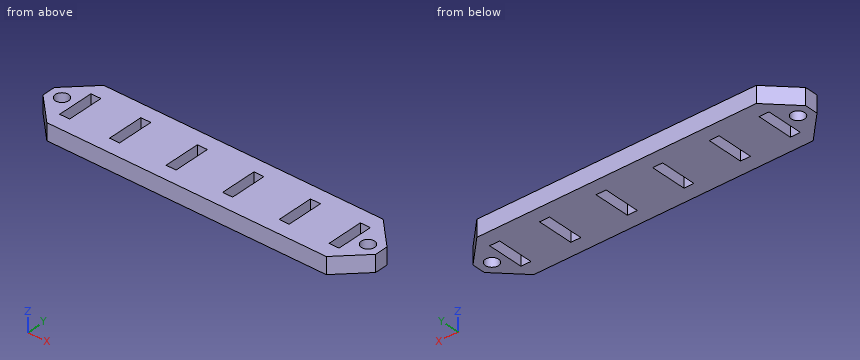
```python
from build123d import *

# Parameters (mm, degrees)
SKETCH1_W           = 100
SKETCH1_H           = 20
BOSS_EXTRUDE1_DEPTH = 5
SKETCH2_R           = 2
SKETCH2_W           = 3
SKETCH2_H           = 11
CUT_EXTRUDE1_DEPTH  = 5
CUT_EXTRUDE2_DEPTH  = 5


with BuildPart() as part:
    # Sketch1 → Boss-Extrude1 (new body)
    with BuildSketch(Plane.XY):
        with Locations((50, 10)):
            Rectangle(SKETCH1_W, SKETCH1_H)
    extrude(amount=BOSS_EXTRUDE1_DEPTH)

    # Sketch2 → Cut-Extrude1 (cut)
    with BuildSketch(Plane(origin=(0, 0, 0), x_dir=(-1, 0, 0), z_dir=(0, 0, -1))):
        with Locations((-96, 10)):
            Circle(SKETCH2_R)
        with Locations((-4, 10)):
            Circle(SKETCH2_R)
        with Locations((-90.5, 10)):
            Rectangle(SKETCH2_W, SKETCH2_H)
        with Locations((-75.5, 10)):
            Rectangle(SKETCH2_W, SKETCH2_H)
        with Locations((-58.5, 10)):
            Rectangle(SKETCH2_W, SKETCH2_H)
        with Locations((-41.5, 10)):
            Rectangle(SKETCH2_W, SKETCH2_H)
        with Locations((-24.5, 10)):
            Rectangle(SKETCH2_W, SKETCH2_H)
        with Locations((-9.5, 10)):
            Rectangle(SKETCH2_W, SKETCH2_H)
    extrude(amount=-CUT_EXTRUDE1_DEPTH, mode=Mode.SUBTRACT)

    # Sketch3 → Cut-Extrude2 (cut)
    with BuildSketch(Plane(origin=(0, 0, 0), x_dir=(-1, 0, 0), z_dir=(0, 0, -1))):
        Polygon((-92, 20), (-100, 12), (-100, 20), align=None)
        Polygon((-100, 8), (-100, 0), (-92, 0), align=None)
        Polygon((-8, 20), (0, 20), (0, 12), align=None)
        Polygon((0, 8), (-8, 0), (0, 0), align=None)
    extrude(amount=-CUT_EXTRUDE2_DEPTH, mode=Mode.SUBTRACT)


solid = part.part
```
For this review, take the finished solid that the model builds, in its own axes (mm). Round coordinates to 2 decimals unless told otherwise and drop trailing zeros. Order: outer loops, then holes, each group sorted by start corner. A loop starts at its lowest first (then second) coordinate and runs counter-clockwise, first axis right, second up.
Q1. We need section A-A, the plane y = 7. Give the boundary of the cut face in (x, z), plus the area to 3 significant figures.
Findings below:
outline: (1, 0) - (8, 0) - (8, 5) - (1, 5) - close; (11, 0) - (23, 0) - (23, 5) - (11, 5) - close; (26, 0) - (40, 0) - (40, 5) - (26, 5) - close; (43, 0) - (57, 0) - (57, 5) - (43, 5) - close; (60, 0) - (74, 0) - (74, 5) - (60, 5) - close; (77, 0) - (89, 0) - (89, 5) - (77, 5) - close; (92, 0) - (99, 0) - (99, 5) - (92, 5) - close
area: 400 mm2
Q2. Insertion check: P1, Ø1, axis at y = 5, z = 1, coming from the +X side. The pin has a flat end and moves straight along its axis. Give the tip position at first contact, or say it passes through.
Findings below:
P1: stops at x = 97.5
Q3. We need section C-C, the plane z = 2.5. State how many separate pieces and enclosed holes the cut face has, plus the area to 3 significant figures.
Findings below:
separate pieces: 1
enclosed holes: 8
area: 1,650 mm2
Q4. We need section D-D, the plane y = 17.5. Give the boundary of the cut face in (x, z).
Findings below:
outline: (5.5, 0) - (94.5, 0) - (94.5, 5) - (5.5, 5) - close
Q5. Wall thickness on line 1 (Y direction, x = 25, z = 3.65); line 2 (Y direction, x = 96, z = 1.75); line 3 (X direction, y = 3.5, z = 0.9): over which ranges is each line inside the solid? List them lowest first.
Findings below:
line 1: y = 0 to 4.5, 15.5 to 20
line 2: y = 4 to 8, 12 to 16
line 3: x = 4.5 to 95.5
Q6. We need section B-B, the plane x = 96. Give the boundary of the cut face in (y, z).
Findings below:
outline: (4, 0) - (8, 0) - (8, 5) - (4, 5) - close; (12, 0) - (16, 0) - (16, 5) - (12, 5) - close
